```python
from build123d import *

# Parameters (mm, degrees)
CROQUIS1_R                  = 3.25
CROQUIS1_R_2                = 2.25
SALIENTE_EXTRUIR1_DEPTH     = 0.8
BRIDA_DE_ARISTA1_DEPTH      = 246
BRIDA_START                 = 0.8
BRIDA_DE_ARISTA1_PROFILE_W  = 246
BRIDA_DE_ARISTA1_PROFILE_H  = 118.4
BRIDA_DE_ARISTA1_PROFILE_R  = 1.5
BRIDA_DE_ARISTA1_FLAT_DEPTH = 0.8


# Sheet-metal steps are written as plain solids
with BuildPart() as part:
    # Croquis1 → Saliente-Extruir1 (new body)
    with BuildSketch(Plane(origin=(0, 0, 0), x_dir=(1, 0, 0), z_dir=(0, 1, 0))):
        Polygon((0, 56), (96, 56), (96, 0), (0, 0), (-150, 0), (-150, 56), align=None)
        with Locations(Location((21, 50, 0), (0, 0, 270))):
            Circle(CROQUIS1_R, mode=Mode.SUBTRACT)
        with Locations(Location((75, 50, 0), (0, 0, 90))):
            Circle(CROQUIS1_R, mode=Mode.SUBTRACT)
        with Locations(Location((75, 6, 0), (0, 0, 270))):
            Circle(CROQUIS1_R, mode=Mode.SUBTRACT)
        with Locations(Location((21, 6, 0), (0, 0, 90))):
            Circle(CROQUIS1_R, mode=Mode.SUBTRACT)
        with Locations(Location((92, 34.25, 0), (0, 0, 270))):
            Circle(CROQUIS1_R_2, mode=Mode.SUBTRACT)
        with Locations(Location((4, 34.25, 0), (0, 0, 90))):
            Circle(CROQUIS1_R_2, mode=Mode.SUBTRACT)
    extrude(amount=SALIENTE_EXTRUIR1_DEPTH)

    # Brida de arista1 bend section (across the edge) → Brida de arista1 (add)
    with BuildSketch(Plane(origin=(-150, 0, -56.8), x_dir=(0, 0, 1), z_dir=(1, 0, 0))):
        with BuildLine():
            Line((-0.8, 0.8), (0, 0.8))
            ThreePointArc((0, 0.8), (0.234314575, 0.234314575), (0.8, 0))
            Line((0.8, 0), (0.8, -0.8))
            ThreePointArc((0.8, -0.8), (-0.33137085, -0.33137085), (-0.8, 0.8))
        make_face()
    extrude(amount=BRIDA_DE_ARISTA1_DEPTH)

    # Brida de arista1 profile (on flange) → Brida de arista1 flat (add)
    with BuildSketch(Plane(origin=(0, 0, -56.8), x_dir=(1, 0, 0), z_dir=(0, 0, -1)).offset(BRIDA_START)):
        with Locations((-27, 60)):
            Rectangle(BRIDA_DE_ARISTA1_PROFILE_W, BRIDA_DE_ARISTA1_PROFILE_H)
        with Locations((22, 9)):
            Circle(BRIDA_DE_ARISTA1_PROFILE_R, mode=Mode.SUBTRACT)
        with Locations((80, 9)):
            Circle(BRIDA_DE_ARISTA1_PROFILE_R, mode=Mode.SUBTRACT)
        with Locations((22, 58)):
            Circle(BRIDA_DE_ARISTA1_PROFILE_R, mode=Mode.SUBTRACT)
        with Locations((80, 58)):
            Circle(BRIDA_DE_ARISTA1_PROFILE_R, mode=Mode.SUBTRACT)
    extrude(amount=-BRIDA_DE_ARISTA1_FLAT_DEPTH)


solid = part.part
```
Geometry check sheet. Reference: the model listing, model coordinates, mm. A direction names the side the tool comes from. Round coordinates to 2 decimals unless told otherwise and drop trailing zeros. Loops run counter-clockwise (first coordinate to the right, second up) from the corner with the lowest first, then second, coordinate; pieces in that order, holes last. Notation, with made-up numbers: (6.25, 54.25) - (63.25, 54.25) arc R16 cw to (63.25, 58.25) - close; hole circle Ø1 at (83, 33). An arc over 180 degrees is marked (long way). Write each question's results on one line, items separated by ' | '. Start each with the question number.
Q1. Thickness scan on line 1 (X direction, y = 0.5, z = -6); line 2 (X direction, y = -9, z = -57.4); line 3 (Y direction, x = 22, z = -57). Record the ranges inside material, lowest first. Write a range as [from, to].
Q2. Release check for a two-part mould opening along Z. For faces 3 (the flat face through (-25, 0.8, -28)), 4 (the flat face through (-29, -61, -56.8)), 5 (the cylindrical face through (20.02, 0.39, -9.1)) record: +Z half, -Z half, draft (parallel to the pull), parting line (faces both ways), or undercut.
Q3. Cross-section at B-B on x = 92. Enter the section's corners in (y, z), and give its area (3 significant figures).
Q4. Cross-section at D-D on z = -49. Enter the section's corners in (x, y), and give its area (3 significant figures).
Q5. Cross-section at C-C on x = -120. Enter the section's corners in (y, z).
Q6. Cross-section at A-A on z = -6. Enter the section's corners in (x, y), and give its area (3 significant figures).
Q7. Gauge pin test, flat ends, axial feed: P1, Ø2, axis at x = -60.5, z = -40, coming from the -Y side; P2, Ø2, axis at x = -120, y = -100.5, coming from the +Z side. Record the tip position at first contact, or that the pin passes through.
Q8. Access from +Z, -Z, +X, -X, +Y, -Y to the whole of each face (thin tool, end or side, straight path). Record for faces 1 (the cylindrical face through (76.245, 0.394, -53.002)), 2 (the flat face through (-25, 0, -28)).
Answers below:
1) line 1: x = [-150, 17.75], [24.25, 71.75], [78.25, 96] | line 2: x = [-150, 20.5], [23.5, 78.5], [81.5, 96] | line 3: y = [-119.2, -59.5], [-56.5, -10.5], [-7.5, 0.45]
2) face 3: draft | face 4: +Z half | face 5: undercut
3) outline: (-119.2, -57.6) - (-0.8, -57.6) arc R1.6 ccw to (0.8, -56) - (0.8, -36.5) - (0, -36.5) - (0, -56) arc R0.8 cw to (-0.8, -56.8) - (-119.2, -56.8) - close; (0, -32) - (0.8, -32) - (0.8, 0) - (0, 0) - close | area: 137 mm²
4) outline: (-150, 0) - (17.91, 0) - (17.91, 0.8) - (-150, 0.8) - close; (24.09, 0) - (71.91, 0) - (71.91, 0.8) - (24.09, 0.8) - close; (78.09, 0) - (96, 0) - (96, 0.8) - (78.09, 0.8) - close | area: 187 mm²
5) outline: (-119.2, -57.6) - (-0.8, -57.6) arc R1.6 ccw to (0.8, -56) - (0.8, 0) - (0, 0) - (0, -56) arc R0.8 cw to (-0.8, -56.8) - (-119.2, -56.8) - close
6) outline: (-150, 0) - (17.75, 0) - (17.75, 0.8) - (-150, 0.8) - close; (24.25, 0) - (71.75, 0) - (71.75, 0.8) - (24.25, 0.8) - close; (78.25, 0) - (96, 0) - (96, 0.8) - (78.25, 0.8) - close | area: 186 mm²
7) P1: stops at y = 0 | P2: stops at z = -56.8
8) face 1: +Y, -Y | face 2: +Z, +X, -X, -Y
